Could you check a few things on this model? Use its own coordinates, in mm. Face numbers are marked on the shaded views. A direction names the side the tool comes from. Give positions to 0.01 mm unless a question says otherwise; leave off trailing zeros. Write each loop counter-clockwise with the first axis right and the second up, starting at its lowest first coordinate (ties: lowest second). Pieces come first, ordered by that corner, then holes. Notation, with made-up numbers: (61.25, 64.25) - (106.25, 64.25) arc R17 cw to (106.25, 92.25) - close; hole circle Ø8 at (52.25, 45.5). An arc over 180 degrees is marked (long way). Use one line per item in the form item = value.
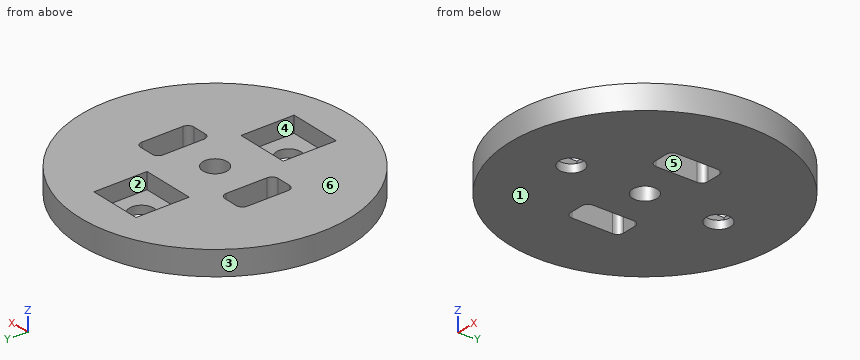
```python
from build123d import *

# Parameters (mm, degrees)
MODEL_R                 = 16.5
MODEL_R_2               = 1.5
SALIENTE_EXTRUIR1_DEPTH = 3
CROQUIS2_W              = 6.5
CROQUIS2_H              = 6.5
CROQUIS2_W_2            = 6.500000001
CORTAR_EXTRUIR1_DEPTH   = 2


with BuildPart() as part:
    # Model → Saliente-Extruir1 (new body)
    with BuildSketch(Plane.XY):
        with Locations((215.747807914, 241.952019993)):
            Circle(MODEL_R)
        with Locations((215.747807914, 241.952019993)):
            Circle(MODEL_R_2, mode=Mode.SUBTRACT)
        with Locations((215.747807914, 232.952019993)):
            Circle(MODEL_R_2, mode=Mode.SUBTRACT)
        with Locations((215.747807914, 250.952019993)):
            Circle(MODEL_R_2, mode=Mode.SUBTRACT)
        with BuildLine():
            Line((223.122807913, 245.202019993), (221.372807913, 245.202019993))
            ThreePointArc((221.372807913, 245.202019993), (220.842477828, 244.982350079), (220.622807913, 244.452019993))
            Line((220.622807913, 244.452019993), (220.622807913, 239.452019993))
            ThreePointArc((220.622807913, 239.452019993), (220.842477828, 238.921689907), (221.372807913, 238.702019993))
            Line((221.372807913, 238.702019993), (223.122807913, 238.702019993))
            ThreePointArc((223.122807913, 238.702019993), (223.653137999, 238.921689907), (223.872807913, 239.452019993))
            Line((223.872807913, 239.452019993), (223.872807913, 244.452019993))
            ThreePointArc((223.872807913, 244.452019993), (223.653137999, 244.982350079), (223.122807913, 245.202019993))
        make_face(mode=Mode.SUBTRACT)
        with BuildLine():
            Line((208.372807913, 245.202019993), (210.122807913, 245.202019993))
            ThreePointArc((210.122807913, 245.202019993), (210.653137999, 244.982350079), (210.872807913, 244.452019993))
            Line((210.872807913, 244.452019993), (210.872807913, 239.452019993))
            ThreePointArc((210.872807913, 239.452019993), (210.653137999, 238.921689907), (210.122807913, 238.702019993))
            Line((210.122807913, 238.702019993), (208.372807913, 238.702019993))
            ThreePointArc((208.372807913, 238.702019993), (207.842477828, 238.921689907), (207.622807913, 239.452019993))
            Line((207.622807913, 239.452019993), (207.622807913, 244.452019993))
            ThreePointArc((207.622807913, 244.452019993), (207.842477828, 244.982350079), (208.372807913, 245.202019993))
        make_face(mode=Mode.SUBTRACT)
    extrude(amount=SALIENTE_EXTRUIR1_DEPTH)

    # Croquis2 → Cortar-Extruir1 (cut)
    with BuildSketch(Plane.XY.offset(3)):
        with Locations((215.747807914, 250.952019993)):
            Rectangle(CROQUIS2_W, CROQUIS2_H)
        with Locations((215.747807914, 232.952019993)):
            Rectangle(CROQUIS2_W_2, CROQUIS2_H)
    extrude(amount=-CORTAR_EXTRUIR1_DEPTH, mode=Mode.SUBTRACT)


solid = part.part
```
1. If I drill on line 1 (X direction, y = 241.5, z = 0.45); line 2 (Z direction, x = 218, y = 253.5); line 3 (X direction, y = 245, z = 0.9), over which ranges is the centre line in solid material (lowest first)? Write a range as from..to.
Response values:
line_1 = 199.25..207.62, 210.87..214.32, 217.18..220.62, 223.87..232.24
line_2 = 0..1
line_3 = 199.53..207.86, 210.63..220.86, 223.63..231.96
2. Imagine slicing it at A-A, the plane z = 2.3. List the corners of the cut face in (x, y) for me, and give its area (3 significant figures).
Response values:
outline = circle Ø33 at (215.75, 241.95); hole (207.62, 239.45) arc R0.75 ccw to (208.37, 238.7) - (210.12, 238.7) arc R0.75 ccw to (210.87, 239.45) - (210.87, 244.45) arc R0.75 ccw to (210.12, 245.2) - (208.37, 245.2) arc R0.75 ccw to (207.62, 244.45) - close; hole (212.5, 229.7) - (219, 229.7) - (219, 236.2) - (212.5, 236.2) - close; hole (212.5, 247.7) - (219, 247.7) - (219, 254.2) - (212.5, 254.2) - close; hole circle Ø3 at (215.75, 241.95); hole (220.62, 239.45) arc R0.75 ccw to (221.37, 238.7) - (223.12, 238.7) arc R0.75 ccw to (223.87, 239.45) - (223.87, 244.45) arc R0.75 ccw to (223.12, 245.2) - (221.37, 245.2) arc R0.75 ccw to (220.62, 244.45) - close
area = 722 mm²
3. Imagine slicing it at C-C, the plane x = 213.5. List the corners of the cut face in (y, z) for me, and give its area (3 significant figures).
Response values:
outline = (225.61, 0) - (258.3, 0) - (258.3, 3) - (254.2, 3) - (254.2, 1) - (247.7, 1) - (247.7, 3) - (236.2, 3) - (236.2, 1) - (229.7, 1) - (229.7, 3) - (225.61, 3) - close
area = 72.1 mm²
4. Imagine slicing it at B-B, the plane y = 240. List the corners of the cut face in (x, z) for me.
Response values:
outline = (199.36, 0) - (207.62, 0) - (207.62, 3) - (199.36, 3) - close; (210.87, 0) - (220.62, 0) - (220.62, 3) - (210.87, 3) - close; (223.87, 0) - (232.13, 0) - (232.13, 3) - (223.87, 3) - close
5. Which directions (+Z, -Z, +X, -X, +Y, -Y) give clear straight access to the entire face, cutting with the end or side of a thin tool? Please do the marked faces 4, 5 and 6.
Response values:
face_4 = +Z
face_5 = +Z, -Z
face_6 = +Z, +X, -X, +Y, -Y
6. For pin 1 (1 mm diameter, centred on y = 252, z = 2, fed in from -X); pin 2 (1.5 mm diameter, centred on y = 240, z = 2.5, fed in from -X); pin 3 (1.5 mm diameter, centred on y = 229.5, z = 2, fed in from -X); pin 4 (5 mm diameter, centred on x = 215, y = 250, fed in from +Z), each with a flat end and sliding along its axis, tell me the tip position at first contact or that it passes through.
Response values:
pin_1 = 202.29
pin_2 = 199.29
pin_3 = 204.12
pin_4 = 3
7. If we mould it in two halves opening along X, with no side actions, what happens to the marked faces 1, 2 and 3? For each: pulls with the +X half, pulls with the -X half, needs draft (parallel to the pull), parting line crosses it, or undercut.
Response values:
face_1 = needs draft
face_2 = undercut
face_3 = parting line crosses it
8. Imagine slicing it at D-D, the plane y = 253. List the corners of the cut face in (x, z) for me.
Response values:
outline = (203.49, 0) - (228, 0) - (228, 3) - (219, 3) - (219, 1) - (212.5, 1) - (212.5, 3) - (203.49, 3) - close
